Can you work these out from the drawing? Everything is in mm from the part's minimum corner. A direction names the side the tool comes from. Round coordinates to 2 decimals unless told otherwise and drop trailing zeros. Write each loop counter-clockwise with the first axis right and the second up, starting at its lowest first coordinate (ties: lowest second). Pieces come first, ordered by that corner, then holes.
Q1. For the marked faces 1 and 2, which set-ups out of +Z, -Z, +X, -X, +Y, -Y let a thin tool reach every point of the face, with its end or its side?
Q2. If we section it at D-D (z = 10.5): Please give me the cut outline in (x, y), plus the area to 3 significant figures.
Q3. If we section it at B-B (x = 6.5): Please give me the cut outline in (y, z).
Q4. I'm going to push flat-ended pins straight in: pin 1 Ø4.5 at (y, z) = (5, 10.5) entering from -X; pin 2 Ø3 at (x, z) = (3, 14.5) entering from +Y; pin 3 Ø3 at (x, z) = (6.5, 37) entering from +Y. Where does each tip first touch, or does it pass through?
Q5. If we section it at A-A (y = 5): Please give me the cut outline in (x, z), plus the area to 3 significant figures.
Q6. Please list where these lines run through material, in increasing order: line 1 along Z through (x, y) = (5, 5); line 2 along Z through (x, y) = (8.5, 6.75); line 3 along Y through (x, z) = (5.5, 10.5).
Q7. If we section it at C-C (z = 22): Please give me the cut outline in (x, y), plus the area to 3 significant figures.
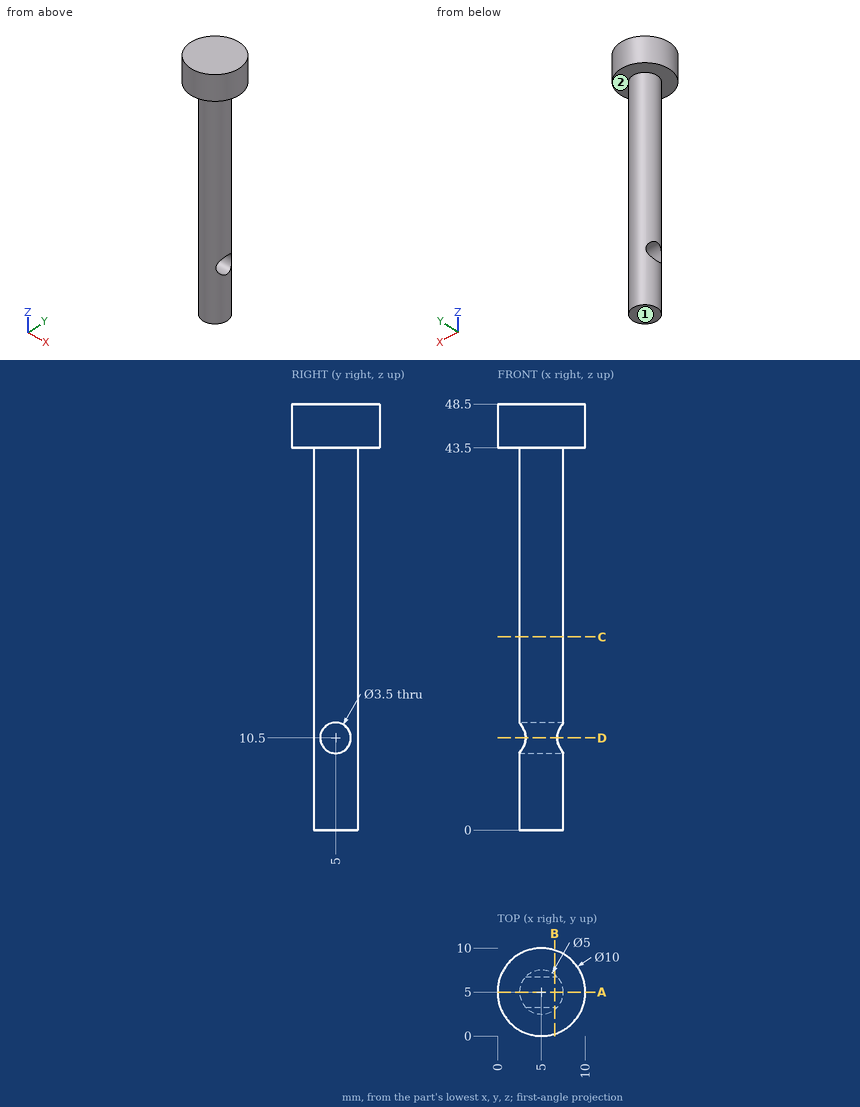
A:
1. face 1: -Z, +X, -X, +Y, -Y
1. face 2: -Z
2. outline: (3.21, 3.25) arc R2.5 ccw to (6.79, 3.25) - close; (3.21, 6.75) - (6.79, 6.75) arc R2.5 ccw to start
2. area: 3.69 mm2
3. outline: (0.23, 43.5) - (3, 43.5) - (3, 0) - (7, 0) - (7, 43.5) - (9.77, 43.5) - (9.77, 48.5) - (0.23, 48.5) - close; hole circle Ø3.5 at (5, 10.5)
4. pin 1: stops at x = 2.5
4. pin 2: stops at y = 7.45
4. pin 3: stops at y = 7.5
5. outline: (0, 43.5) - (2.5, 43.5) - (2.5, 12.25) - (7.5, 12.25) - (7.5, 43.5) - (10, 43.5) - (10, 48.5) - (0, 48.5) - close; (2.5, 0) - (7.5, 0) - (7.5, 8.75) - (2.5, 8.75) - close
5. area: 250 mm2
6. line 1: z = 0 to 8.75, 12.25 to 48.5
6. line 2: z = 43.5 to 48.5
6. line 3: y = 2.55 to 3.25, 6.75 to 7.45
7. outline: circle Ø5 at (5, 5)
7. area: 19.6 mm2
